Could you check a few things on this model? Use its own coordinates, in mm. A direction names the side the tool comes from. Round coordinates to 2 decimals unless told otherwise and drop trailing zeros. Order: outer loops, then holes, each group sorted by start corner. A loop starts at its lowest first (then second) coordinate and runs counter-clockwise, first axis right, second up. Notation, with made-up numbers: (-20, 73) - (26, 73) arc R19 cw to (26, 108) - close; hole circle Ø3 at (8.25, 28.5). An arc over 180 degrees is marked (long way). Use one line per item in the form item = value.
from build123d import *

# Parameters (mm, degrees)
BOSS_EXTRUDE1_DEPTH = 10
BOSS_EXTRUDE2_START = -2
BOSS_EXTRUDE2_DEPTH = 2
BOSS_EXTRUDE3_DEPTH = 2
SKETCH6_R           = 4.5
SKETCH6_R_2         = 2.9
BOSS_EXTRUDE4_DEPTH = 25
CUT_EXTRUDE1_START  = -8
SKETCH7_R           = 2.9
CUT_EXTRUDE1_DEPTH  = 8
SKETCH9_R           = 2.5
BOSS_EXTRUDE5_DEPTH = 10
BOSS_EXTRUDE6_START = -25
BOSS_EXTRUDE6_DEPTH = 25
SKETCH13_W          = 16.297841409
SKETCH13_H          = 10
BOSS_EXTRUDE7_DEPTH = 15
SKETCH14_W          = 6
SKETCH14_H          = 4.2
CUT_EXTRUDE4_DEPTH  = 8
SKETCH17_W          = 10
SKETCH17_H          = 0.143122073
CUT_EXTRUDE5_DEPTH  = 16.297841409
SKETCH18_R          = 3
CUT_EXTRUDE6_DEPTH  = 3


with BuildPart() as part:
    # Sketch1 → Boss-Extrude1 (new body)
    with BuildSketch(Plane.XY):
        with BuildLine():
            Line((0, 0), (0, 15))
            Line((0, 15), (38.500664221, 14.856877927))
            Line((38.500664221, 14.856877927), (42, 18.580686342))
            Line((42, 18.580686342), (47, 18.580686342))
            Line((47, 18.580686342), (52, 18.580686342))
            Line((52, 18.580686342), (55.499335779, 14.856877927))
            Line((55.499335779, 14.856877927), (80.635168579, 14.856877927))
            Line((80.635168579, 14.856877927), (84.134504358, 18.580686342))
            Line((84.134504358, 18.580686342), (89.134504358, 18.580686342))
            Line((89.134504358, 18.580686342), (94.134504358, 18.580686342))
            Line((94.134504358, 18.580686342), (97.633840137, 14.856877927))
            Line((97.633840137, 14.856877927), (136.134504358, 14.856877927))
            Line((136.134504358, 14.856877927), (136.134504358, 0))
            Line((136.134504358, 0), (96.134504358, 0))
            ThreePointArc((96.134504358, 0), (89.134504358, 7), (82.134504358, 0))
            Line((82.134504358, 0), (54, 0))
            ThreePointArc((54, 0), (47, 7), (40, 0))
            Line((40, 0), (0, 0))
        make_face()
        with BuildLine():
            Line((81.500231462, 12.856877927), (54.634272896, 12.856877927))
            Line((54.634272896, 12.856877927), (51.134937117, 16.580686342))
            Line((51.134937117, 16.580686342), (47, 16.580686342))
            Line((47, 16.580686342), (42.865062883, 16.580686342))
            Line((42.865062883, 16.580686342), (39.365727104, 12.856877927))
            Line((39.365727104, 12.856877927), (2, 12.856877927))
            Line((2, 12.856877927), (2, 2))
            Line((2, 2), (38.225035613, 2))
            ThreePointArc((38.225035613, 2), (47, 9), (55.774964387, 2))
            Line((55.774964387, 2), (80.35953997, 2))
            ThreePointArc((80.35953997, 2), (89.134504358, 9), (97.909468745, 2))
            Line((97.909468745, 2), (134.134504358, 2))
            Line((134.134504358, 2), (134.134504358, 12.856877927))
            Line((134.134504358, 12.856877927), (96.768777254, 12.856877927))
            Line((96.768777254, 12.856877927), (93.269441475, 16.580686342))
            Line((93.269441475, 16.580686342), (89.134504358, 16.580686342))
            Line((89.134504358, 16.580686342), (84.999567241, 16.580686342))
            Line((84.999567241, 16.580686342), (81.500231462, 12.856877927))
        make_face(mode=Mode.SUBTRACT)
    extrude(amount=BOSS_EXTRUDE1_DEPTH)

    # Sketch2 → Boss-Extrude2 (add)
    with BuildSketch(Plane.XY.offset(10).offset(BOSS_EXTRUDE2_START)):
        with BuildLine():
            Line((136.134504358, 0), (136.134504358, 14.856877927))
            Line((136.134504358, 14.856877927), (97.633840137, 14.856877927))
            Line((97.633840137, 14.856877927), (94.134504358, 18.580686342))
            Line((94.134504358, 18.580686342), (84.134504358, 18.580686342))
            Line((84.134504358, 18.580686342), (80.635168579, 14.856877927))
            Line((80.635168579, 14.856877927), (55.499335779, 14.856877927))
            Line((55.499335779, 14.856877927), (52, 18.580686342))
            Line((52, 18.580686342), (42, 18.580686342))
            Line((42, 18.580686342), (38.500664221, 14.856877927))
            Line((38.500664221, 14.856877927), (0, 15))
            Line((0, 15), (0, 0))
            Line((0, 0), (40, 0))
            ThreePointArc((40, 0), (47, 7), (54, 0))
            Line((54, 0), (82.134504358, 0))
            ThreePointArc((82.134504358, 0), (89.134504358, 7), (96.134504358, 0))
            Line((96.134504358, 0), (136.134504358, 0))
        make_face()
    extrude(amount=BOSS_EXTRUDE2_DEPTH)

    # Sketch3 → Boss-Extrude3 (add)
    with BuildSketch(Plane(origin=(0, 0, 0), x_dir=(-1, 0, 0), z_dir=(0, 0, -1))):
        with BuildLine():
            Line((0, 15), (-38.500664221, 14.856877927))
            Line((-38.500664221, 14.856877927), (-42, 18.580686342))
            Line((-42, 18.580686342), (-52, 18.580686342))
            Line((-52, 18.580686342), (-55.499335779, 14.856877927))
            Line((-55.499335779, 14.856877927), (-80.635168579, 14.856877927))
            Line((-80.635168579, 14.856877927), (-84.134504358, 18.580686342))
            Line((-84.134504358, 18.580686342), (-94.134504358, 18.580686342))
            Line((-94.134504358, 18.580686342), (-97.633840137, 14.856877927))
            Line((-97.633840137, 14.856877927), (-136.134504358, 14.856877927))
            Line((-136.134504358, 14.856877927), (-136.134504358, 0))
            Line((-136.134504358, 0), (-96.134504358, 0))
            ThreePointArc((-96.134504358, 0), (-89.134504358, 7), (-82.134504358, 0))
            Line((-82.134504358, 0), (-54, 0))
            ThreePointArc((-54, 0), (-47, 7), (-40, 0))
            Line((-40, 0), (0, 0))
            Line((0, 0), (0, 15))
        make_face()
    extrude(amount=-BOSS_EXTRUDE3_DEPTH)

    # Sketch6 → Boss-Extrude4 (add)
    with BuildSketch(Plane.XY.offset(10)):
        with Locations(Location((68.134504358, 7.717300047, 0), (0, 0, 180))):
            Circle(SKETCH6_R)
        with Locations((68.134504358, 7.717300047)):
            Circle(SKETCH6_R_2, mode=Mode.SUBTRACT)
    extrude(amount=BOSS_EXTRUDE4_DEPTH)

    # Sketch7 → Cut-Extrude1 (cut)
    with BuildSketch(Plane.XY.offset(10).offset(CUT_EXTRUDE1_START)):
        with Locations((68.134504358, 7.717300047)):
            Circle(SKETCH7_R)
    extrude(amount=CUT_EXTRUDE1_DEPTH, mode=Mode.SUBTRACT)

    # Sketch9 → Boss-Extrude5 (add)
    with BuildSketch(Plane.XY.offset(10)):
        with Locations((126.134504358, 7.356877927)):
            Circle(SKETCH9_R)
        with Locations((103, 7.5)):
            Circle(SKETCH9_R)
        with Locations((80.134504358, 7.5)):
            Circle(SKETCH9_R)
        with Locations((10.134504358, 7.356877927)):
            Circle(SKETCH9_R)
        with Locations((33.269008716, 7.5)):
            Circle(SKETCH9_R)
        with Locations((56.134504358, 7.5)):
            Circle(SKETCH9_R)
    extrude(amount=-BOSS_EXTRUDE5_DEPTH)

    # Sketch10 → Boss-Extrude6 (add)
    with BuildSketch(Plane.XY.offset(35).offset(BOSS_EXTRUDE6_START)):
        with BuildLine():
            Line((63.634504358, 7.717300047), (63.634504358, 0))
            Line((63.634504358, 0), (72.634504358, 0))
            Line((72.634504358, 0), (72.634504358, 7.717300047))
            ThreePointArc((72.634504358, 7.717300047), (68.134504358, 3.217300047), (63.634504358, 7.717300047))
        make_face()
    extrude(amount=BOSS_EXTRUDE6_DEPTH)

    # Sketch13 → Boss-Extrude7 (add)
    with BuildSketch(Plane.XZ):
        with Locations((8.148920705, 5)):
            Rectangle(SKETCH13_W, SKETCH13_H)
        with Locations((128.120088012, 5)):
            Rectangle(SKETCH13_W, SKETCH13_H)
    extrude(amount=-BOSS_EXTRUDE7_DEPTH)

    # Sketch14 → Cut-Extrude4 (cut)
    with BuildSketch(Plane.XZ):
        with Locations((12, 5)):
            Rectangle(SKETCH14_W, SKETCH14_H)
        with Locations((124.269008716, 5)):
            Rectangle(SKETCH14_W, SKETCH14_H)
    extrude(amount=-CUT_EXTRUDE4_DEPTH, mode=Mode.SUBTRACT)

    # Sketch17 → Cut-Extrude5 (cut)
    with BuildSketch(Plane.ZY.offset(-119.971167307)):
        with Locations((5, 14.928438964)):
            Rectangle(SKETCH17_W, SKETCH17_H)
    extrude(amount=-CUT_EXTRUDE5_DEPTH, mode=Mode.SUBTRACT)

    # Sketch18 → Cut-Extrude6 (cut)
    with BuildSketch(Plane(origin=(0, 0, 0), x_dir=(-1, 0, 0), z_dir=(0, 0, -1))):
        with Locations((-116.201756537, 7.428438964)):
            Circle(SKETCH18_R)
        with Locations((-19.932747821, 7.428438964)):
            Circle(SKETCH18_R)
    extrude(amount=-CUT_EXTRUDE6_DEPTH, mode=Mode.SUBTRACT)


solid = part.part
Item 1: If we mould it in two halves opening along Y, with no side actions, what happens to faces 1 (the face through (118.58, 5.6, 0.99)), 2 (the face through (47, 7, 5)), 3 (the face through (12, 4, 2.9)), 4 (the face through (47, 9, 5))? For each: released by +Y, released by -Y, zero draft, split by the parting line, or undercut.
Found:
face_1 = undercut
face_2 = released by -Y
face_3 = zero draft
face_4 = undercut
Item 2: I need wall thicknesses on L1, parallel to Z at x = 30, y = 8.5; L2, parallel to X at y = 8.75, z = 19.5; L3, parallel to Y at x = 78.5, z = 9. Which ranges of each line are inside material? Lowest first, please.
Found:
L1 = 0 to 2, 8 to 10
L2 = 63.75 to 65.42, 70.84 to 72.51
L3 = 0 to 14.86
Item 3: Imagine slicing it at C-C on z = 15. Please give me the cut outline in (x, y).
Found:
outline = (63.63, 0) - (72.63, 0) - (72.63, 7.72) arc R4.5 ccw to (63.63, 7.72) - close; hole circle Ø5.8 at (68.13, 7.72)
Item 4: Imagine slicing it at A-A on x = 103. Please give me the cut outline in (y, z).
Found:
outline = (0, 0) - (14.86, 0) - (14.86, 10) - (0, 10) - close; hole (2, 2) - (5, 2) - (5, 8) - (2, 8) - close; hole (10, 2) - (12.86, 2) - (12.86, 8) - (10, 8) - close
Item 5: Imagine slicing it at B-B on x = 47. Please give me the cut outline in (y, z).
Found:
outline = (7, 0) - (18.58, 0) - (18.58, 10) - (7, 10) - close; hole (9, 2) - (16.58, 2) - (16.58, 8) - (9, 8) - close
Item 6: For faces 5 (the face through (12, 4, 7.1)), 6 (the face through (67.1, 4.8, 35)), 7 (the face through (8, 15, 5)), 8 (the face through (47, 16.581, 5)), 9 (the face through (53.73, 16.74, 4.93)), which set-ups out of +Z, -Z, +X, -X, +Y, -Y let a thin tool reach every point of the face, with its end or its side?
Found:
face_5 = -Y
face_6 = +Z, +X, -X, +Y, -Y
face_7 = +Z, -Z, -X, +Y
face_8 = none
face_9 = +Z, -Z, +Y
Item 7: Will these pins go through, and if not, where does the flat tip stop? P1, Ø1.8, axis at x = 109, z = 5.5, coming from the +Y side; P2, Ø8, axis at x = 6.5, z = 3, coming from the +Y side; P3, Ø5.5, axis at x = 116.2, y = 7.43, coming from the -Z side.
Found:
P1 = 14.86
P2 = 15
P3 = 8
